Part model, mm, in its own coordinate system. Face numbers are marked on the shaded views. A direction names the side the tool comes from. Give positions to 0.01 mm unless a question says otherwise; leave off trailing zeros. Write each loop counter-clockwise with the first axis right and the second up, starting at its lowest first coordinate (ties: lowest second). Pieces come first, ordered by that corner, then holes. Notation, with made-up numbers: M 35.5,64.25 L 46.5,64.25 A13 ccw 46.5,80.25 Z; hole C -6,15.25 d2. An arc over 180 degrees is marked long. Use CSV: the item, a comma, the result in double quotes. Start each with the question number.
1. Band-saw the part on C-C, the plane x = 10.5. List the corners of the cut face in (y, z).
2. Band-saw the part on B-B, the plane x = 6.45. List the corners of the cut face in (y, z), then the cut area to 3 significant figures.
3. Band-saw the part on D-D, the plane y = 6.75. List the corners of the cut face in (x, z).
4. Band-saw the part on A-A, the plane z = -6.5. List the corners of the cut face in (x, y), then the cut area to 3 significant figures.
5. Mould opens along Y. For the marked faces 4, 5 and 6 say: pulls with the +Y half, pulls with the -Y half, needs draft (parallel to the pull), parting line crosses it, or undercut.
6. Drill centre lines: line 1 along Z through (x, y) = (11.5, 12.25); line 2 along Y through (x, z) = (12.25, -9.75); line 3 along Z through (x, y) = (7, 1). Where is each one in solid material? Low to high. Write a range as from..to.
7. 3-axis set-ups, long thin cutter, end or side, ignore diameter. For the marked faces 1, 2 and 3: which of +Z, -Z, +X, -X, +Y, -Y reach the whole face in a straight line?
8. Drop flat-ended pins along their axis: pin 1 Ø4 at (x, y) = (10, 13) entering from +Z; pin 2 Ø5 at (x, y) = (7.5, 5.5) entering from -Z; pin 3 Ø5 at (x, y) = (7, 6.5) entering from +Z. Give the stop position or say it passes through.
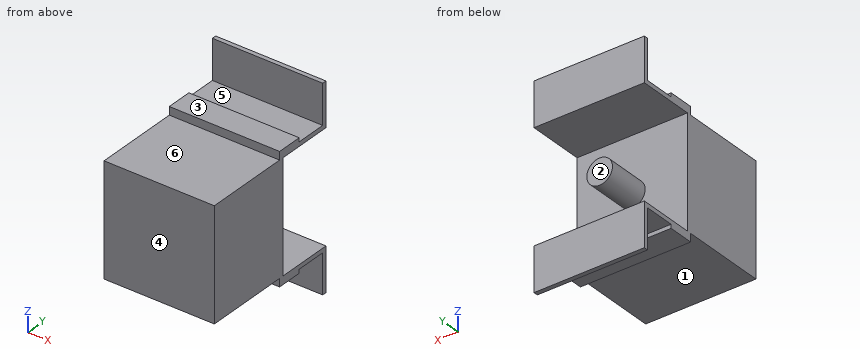
from build123d import *

# Parameters (mm, degrees)
SKETCH1_W           = 12.9
SKETCH1_H           = 13
BOSS_EXTRUDE1_DEPTH = 10
BOSS_EXTRUDE2_DEPTH = 12.9
SKETCH3_W           = 0.45
SKETCH3_H           = 3
BOSS_EXTRUDE3_DEPTH = 12.9
SKETCH4_R           = 1.5
BOSS_EXTRUDE4_DEPTH = 5


with BuildPart() as part:
    # Sketch1 → Boss-Extrude1 (new body)
    with BuildSketch(Plane(origin=(0, 0, 0), x_dir=(1, 0, 0), z_dir=(0, 1, 0))):
        with Locations((6.45, 6.5)):
            Rectangle(SKETCH1_W, SKETCH1_H)
    extrude(amount=BOSS_EXTRUDE1_DEPTH)

    # Sketch2 → Boss-Extrude2 (add)
    with BuildSketch(Plane(origin=(12.9, 0, 0), x_dir=(0, 0, -1), z_dir=(1, 0, 0))):
        Polygon((6.5, 10), (6.5, 10.5), (0, 10.5), (0, 17.1), (-5.135999104, 17.1), (-5.135999104, 16.6), (-0.5, 16.6), (-0.5, 10), (0, 10), align=None)
        Polygon((13, 17.1), (13, 10.5), (6.5, 10.5), (6.5, 10), (13, 10), (13.5, 10), (13.5, 16.6), (18.135999104, 16.6), (18.135999104, 17.1), align=None)
    extrude(amount=-BOSS_EXTRUDE2_DEPTH)

    # Sketch3 → Boss-Extrude3 (add)
    with BuildSketch(Plane(origin=(12.9, 0, 0), x_dir=(0, 0, -1), z_dir=(1, 0, 0))):
        with Locations((-0.725, 11.5)):
            Rectangle(SKETCH3_W, SKETCH3_H)
        with Locations((13.725, 11.5)):
            Rectangle(SKETCH3_W, SKETCH3_H)
    extrude(amount=-BOSS_EXTRUDE3_DEPTH)

    # Sketch4 → Boss-Extrude4 (add)
    with BuildSketch(Plane(origin=(0, 10.5, 0), x_dir=(1, 0, 0), z_dir=(0, 1, 0))):
        with Locations(Location((6.45, 6.5, 0), (0, 0, 90))):
            Circle(SKETCH4_R)
    extrude(amount=BOSS_EXTRUDE4_DEPTH)


solid = part.part
Output:
1,outline,"M 0,-13 L 10,-13 L 10,-13.95 L 13,-13.95 L 13,-13.5 L 16.6,-13.5 L 16.6,-18.14 L 17.1,-18.14 L 17.1,-13 L 10.5,-13 L 10.5,0 L 17.1,0 L 17.1,5.14 L 16.6,5.14 L 16.6,0.5 L 13,0.5 L 13,0.95 L 10,0.95 L 10,0 L 0,0 Z"
2,outline,"M 0,-13 L 10,-13 L 10,-13.95 L 13,-13.95 L 13,-13.5 L 16.6,-13.5 L 16.6,-18.14 L 17.1,-18.14 L 17.1,-13 L 10.5,-13 L 10.5,-8 L 15.5,-8 L 15.5,-5 L 10.5,-5 L 10.5,0 L 17.1,0 L 17.1,5.14 L 16.6,5.14 L 16.6,0.5 L 13,0.5 L 13,0.95 L 10,0.95 L 10,0 L 0,0 Z"
2,area,"166 mm²"
3,outline,"M 0,-13 L 12.9,-13 L 12.9,0 L 0,0 Z"
4,outline,"M 0,0 L 12.9,0 L 12.9,10.5 L 7.95,10.5 L 7.95,15.5 L 4.95,15.5 L 4.95,10.5 L 0,10.5 Z"
4,area,"150 mm²"
5,face 4,"pulls with the -Y half"
5,face 5,"undercut"
5,face 6,"needs draft"
6,line 1,"z = -13.95..-13, 0..0.95"
6,line 2,"y = 0..10.5"
6,line 3,"z = -13..0"
7,face 1,"-Z, +X, -X, -Y"
7,face 2,"+X, -X, +Y"
7,face 3,"+Z, +X, -X, -Y"
8,pin 1,"stops at z = 0.95"
8,pin 2,"stops at z = -13"
8,pin 3,"stops at z = 0"
